from build123d import *

# Parameters (mm, degrees)
SKETCH2_R               = 10.5
BOSS_EXTRUDE1_DEPTH     = 40
SKETCH4_W               = 14
SKETCH4_H               = 22
BOSS_EXTRUDE2_DEPTH     = 38
CUT_EXTRUDE1_DEPTH      = 49.890183064
CUT_EXTRUDE1_DEPTH_BACK = 49.890183064
SKETCH5_W               = 28
SKETCH5_H               = 32.5
SKETCH6_W               = 14
SKETCH6_H               = 38
BOSS_EXTRUDE3_DEPTH     = 40
SKETCH7_W               = 9.5
SKETCH7_H               = 25
BOSS_EXTRUDE4_DEPTH     = 14
BOSS_EXTRUDE5_DEPTH     = 14
SKETCH9_W               = 1
SKETCH9_H               = 30
SKETCH9_H_2             = 31
SKETCH9_H_3             = 20
SKETCH9_H_4             = 15
CUT_EXTRUDE2_DEPTH      = 1
FILLET1_R               = 5
SKETCH10_R              = 12.5
CUT_EXTRUDE3_DEPTH      = 6
SKETCH11_R              = 2.05
CUT_EXTRUDE4_DEPTH      = 116.062756142
SKETCH12_R              = 6
CUT_EXTRUDE5_DEPTH      = 5
CUT_EXTRUDE6_REACH      = 112.061
SKETCH13_R              = 2.05
SKETCH14_R              = 4.5
CUT_EXTRUDE7_DEPTH      = 2
SKETCH15_R              = 1.05
CUT_EXTRUDE8_DEPTH      = 112.975166224
SKETCH17_R              = 2
CUT_EXTRUDE9_DEPTH      = 4


with BuildPart() as part:
    # Sketch2 → Boss-Extrude1 (new body)
    with BuildSketch(Plane.XY):
        Circle(SKETCH2_R)
    extrude(amount=BOSS_EXTRUDE1_DEPTH)

    # Sketch4 → Boss-Extrude2 (add)
    with BuildSketch(Plane.XY.offset(40)):
        with Locations((0, 11)):
            Rectangle(SKETCH4_W, SKETCH4_H)
    extrude(amount=-BOSS_EXTRUDE2_DEPTH)

    # Sketch5 → Cut-Extrude1 (cut, two sides: drawn at the far end of the back side and taken through both)
    with BuildSketch(Plane(origin=(7, 0, 0), x_dir=(0, 0, -1), z_dir=(1, 0, 0)).offset(-CUT_EXTRUDE1_DEPTH_BACK)):
        with Locations((-21, 5.75)):
            Rectangle(SKETCH5_W, SKETCH5_H)
    extrude(amount=CUT_EXTRUDE1_DEPTH + CUT_EXTRUDE1_DEPTH_BACK, mode=Mode.SUBTRACT)


with BuildPart() as cut_extrude1_piece_1:
    # of the separate pieces the step leaves, piece 1, a body of its own (cut_extrude1_pieces)
    add(part.part.solids().sort_by_distance((10.5, 0, 0))[0])



with BuildPart() as cut_extrude1_piece_2:
    # of the separate pieces the step leaves, piece 2, a body of its own (cut_extrude1_pieces)
    add(part.part.solids().sort_by_distance((7, 7.826237921, 40))[0])


with BuildPart() as cut_extrude1_piece_1_1:
    add(cut_extrude1_piece_1.part)

    add(cut_extrude1_piece_2.part)  # Boss-Extrude3 merges Cut-Extrude1 piece 2
    # Sketch6 → Boss-Extrude3 (add)
    with BuildSketch(Plane(origin=(0, 22, 0), x_dir=(1, 0, 0), z_dir=(0, 1, 0))):
        with Locations((0, -21)):
            Rectangle(SKETCH6_W, SKETCH6_H)
    extrude(amount=BOSS_EXTRUDE3_DEPTH)

    # Sketch7 → Boss-Extrude4 (add)
    with BuildSketch(Plane(origin=(7, 0, 0), x_dir=(0, 0, -1), z_dir=(1, 0, 0))):
        Polygon((-52, 42), (-40, 42), (-40, 62), (-40, 67), (-52, 67), align=None)
        Polygon((-40, 67), (-40, 62), (-30.5, 62), (-30.5, 97), (-40, 97), align=None)
        Polygon((-30.5, 97), (-30.5, 62), (-21, 62), (-21, 98), (-21, 102), (-30.5, 102), align=None)
        Polygon((-21, 98), (-21, 62), (-11.5, 62), (-11.5, 87), (-11.5, 98), align=None)
        with Locations((-6.75, 74.5)):
            Rectangle(SKETCH7_W, SKETCH7_H)
    extrude(amount=-BOSS_EXTRUDE4_DEPTH)

    # Sketch8 → Boss-Extrude5 (add)
    with BuildSketch(Plane(origin=(7, 0, 0), x_dir=(0, 0, -1), z_dir=(1, 0, 0))):
        Polygon((-52, 42), (-40, 30), (-40, 42), align=None)
    extrude(amount=-BOSS_EXTRUDE5_DEPTH)

    # Sketch9 → Cut-Extrude2 (cut)
    with BuildSketch(Plane(origin=(7, 0, 0), x_dir=(0, 0, -1), z_dir=(1, 0, 0))):
        with Locations((-30.5, 82)):
            Rectangle(SKETCH9_W, SKETCH9_H)
        with Locations((-21, 82.5)):
            Rectangle(SKETCH9_W, SKETCH9_H_2)
        with Locations((-11.5, 77)):
            Rectangle(SKETCH9_W, SKETCH9_H_3)
        with Locations((-40, 59.5)):
            Rectangle(SKETCH9_W, SKETCH9_H_4)
    extrude(amount=-CUT_EXTRUDE2_DEPTH, mode=Mode.SUBTRACT)

    # Fillet1
    # the kernel refuses this fillet: 5 mm, written as the material it takes off along each edge
    with BuildSketch(Plane(origin=(19.5, 67, 52), x_dir=(0, -1, 0), z_dir=(-1, 0, 0)), Plane(origin=(19.5, 97, 40), x_dir=(0, -1, 0), z_dir=(-1, 0, 0)), Plane(origin=(19.5, 102, 30.5), x_dir=(0, -1, 0), z_dir=(-1, 0, 0)), Plane(origin=(19.5, 98, 11.5), x_dir=(0, 0, 1), z_dir=(-1, 0, 0)), Plane(origin=(19.5, 87, 2), x_dir=(0, 0, 1), z_dir=(-1, 0, 0))) as fillet1_piece_1:
        with BuildLine():
            CenterArc((FILLET1_R, -FILLET1_R), FILLET1_R, 90, 90)
            Line((0, -FILLET1_R), (-FILLET1_R * 0.02, -FILLET1_R))
            Line((-FILLET1_R * 0.02, -FILLET1_R), (-FILLET1_R * 0.02, FILLET1_R * 0.02))
            Line((-FILLET1_R * 0.02, FILLET1_R * 0.02), (FILLET1_R, FILLET1_R * 0.02))
            Line((FILLET1_R, FILLET1_R * 0.02), (FILLET1_R, 0))
        make_face()
    extrude(amount=39, mode=Mode.SUBTRACT)
    with BuildSketch(Plane(origin=(19.247448714, 102, 21), x_dir=(0, 0, 1), z_dir=(-1, 0, 0))) as fillet1_piece_2:
        with BuildLine():
            CenterArc((4.898979486, -5), FILLET1_R, 90, 78.463040967)
            Line((0, -4), (-0.09797959, -3.98))
            ThreePointArc((-0.09797959, -3.98), (-0.1, -2), (-0.1, 0))
            Line((-0.1, 0), (0, 0.1))
            Line((0, 0.1), (4.898979486, 0.1))
            Line((4.898979486, 0.1), (4.898979486, 0))
        make_face()
    extrude(amount=38.494897428, mode=Mode.SUBTRACT)

    # Sketch10 → Cut-Extrude3 (cut)
    with BuildSketch(Plane.ZY.offset(7)):
        with Locations((21, 52)):
            Circle(SKETCH10_R)
    extrude(amount=-CUT_EXTRUDE3_DEPTH, mode=Mode.SUBTRACT)

    # Sketch11 → Cut-Extrude4 (cut, through all)
    with BuildSketch(Plane.ZY.offset(1)):
        with Locations((21, 52)):
            Circle(SKETCH11_R)
    extrude(amount=-CUT_EXTRUDE4_DEPTH, mode=Mode.SUBTRACT)

    # Sketch12 → Cut-Extrude5 (cut)
    with BuildSketch(Plane(origin=(7, 0, 0), x_dir=(0, 0, -1), z_dir=(1, 0, 0))):
        with Locations(Location((-21, 52, 0), (0, 0, 90))):
            Circle(SKETCH12_R)
    extrude(amount=-CUT_EXTRUDE5_DEPTH, mode=Mode.SUBTRACT)

    # Sketch13 → Cut-Extrude6 (cut, up to next)
    with BuildSketch(Plane.XY.offset(40), mode=Mode.PRIVATE) as cut_extrude6_sk1:
        Circle(SKETCH13_R)
    cut_extrude6_tool1 = extrude(cut_extrude6_sk1.sketch, amount=-CUT_EXTRUDE6_REACH, mode=Mode.PRIVATE) & cut_extrude1_piece_1_1.part
    add(cut_extrude6_tool1.solids().sort_by_distance((0, 0, 40))[0], mode=Mode.SUBTRACT)

    # Sketch14 → Cut-Extrude7 (cut)
    with BuildSketch(Plane(origin=(0, 0, 35), x_dir=(-1, 0, 0), z_dir=(0, 0, -1))):
        with Locations(Location((0, 0, 0), (0, 0, 90))):
            Circle(SKETCH14_R)
    extrude(amount=-CUT_EXTRUDE7_DEPTH, mode=Mode.SUBTRACT)

    # Sketch15 → Cut-Extrude8 (cut, through all)
    with BuildSketch(Plane.XY.offset(7)):
        with Locations((-6.062177826, 3.5)):
            Circle(SKETCH15_R)
        with Locations((-6.062177826, -3.5)):
            Circle(SKETCH15_R)
        with Locations((-3.5, -6.062177826)):
            Circle(SKETCH15_R)
        with Locations((0, -7)):
            Circle(SKETCH15_R)
        with Locations((3.5, -6.062177826)):
            Circle(SKETCH15_R)
        with Locations((6.062177826, -3.5)):
            Circle(SKETCH15_R)
        with Locations((7, 0)):
            Circle(SKETCH15_R)
        with Locations((6.062177826, 3.5)):
            Circle(SKETCH15_R)
        with Locations((3.5, 6.062177826)):
            Circle(SKETCH15_R)
        with Locations((0, 7)):
            Circle(SKETCH15_R)
        with Locations((-3.5, 6.062177826)):
            Circle(SKETCH15_R)
        with Locations((-7, 0)):
            Circle(SKETCH15_R)
    extrude(amount=-CUT_EXTRUDE8_DEPTH, mode=Mode.SUBTRACT)

    # Sketch17 → Cut-Extrude9 (cut)
    with BuildSketch(Plane.XY.offset(7)):
        with Locations((0, 7)):
            Circle(SKETCH17_R)
        with Locations((3.5, 6.062177826)):
            Circle(SKETCH17_R)
        with Locations((-3.5, 6.062177826)):
            Circle(SKETCH17_R)
        with Locations((-6.062177826, 3.5)):
            Circle(SKETCH17_R)
        with Locations((-7, 0)):
            Circle(SKETCH17_R)
        with Locations((-6.062177826, -3.5)):
            Circle(SKETCH17_R)
        with Locations((-3.5, -6.062177826)):
            Circle(SKETCH17_R)
        with Locations((0, -7)):
            Circle(SKETCH17_R)
        with Locations((3.5, -6.062177826)):
            Circle(SKETCH17_R)
        with Locations((6.062177826, -3.5)):
            Circle(SKETCH17_R)
        with Locations((7, 0)):
            Circle(SKETCH17_R)
        with Locations((6.062177826, 3.5)):
            Circle(SKETCH17_R)
    extrude(amount=-CUT_EXTRUDE9_DEPTH, mode=Mode.SUBTRACT)


solid = cut_extrude1_piece_1_1.part
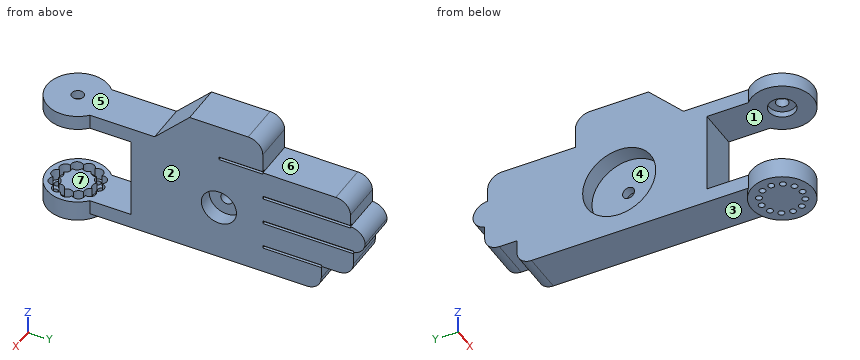
For this review, take the finished solid that the model builds, in its own axes (mm). Face numbers are marked on the shaded views. A direction names the side the tool comes from. Coordinates: 2 decimals unless noted, no trailing zeros. Loops run counter-clockwise (first coordinate to the right, second up) from the corner with the lowest first, then second, coordinate; pieces in that order, holes last. Notation, with made-up numbers: (19.5, -12) -> (65.5, -12) arc R18 ccw to (65.5, 4) -> close; hole circle Ø6 at (22, -21.75). An arc over 180 degrees is marked (long way). Write each question's results on one line, items separated by ' | '.
Q1. Mouldability with a two-part tool opening along Z and no side actions: class the marked faces 1, 2 and 3 as +Z half, -Z half, draft (parallel to the pull), parting line (faces both ways), or undercut.
Taken from the geometry:
face 1: undercut | face 2: draft | face 3: -Z half
Q2. Add section C-C, the plane y = 33. State the section outline as (x, z) points.
Taken from the geometry:
outline: (-7, 2) -> (7, 2) -> (7, 43) -> (-7, 43) -> close
Q3. To check wall thickness, follow line 1 along Z through (x, y) = (4.5, 16); line 2 along Z through (x, y) = (-3, 5); line 3 along Y through (x, z) = (-3.5, 22). State the ranges of each line that lie inside material, in increasing order. Write a range as [from, to].
Taken from the geometry:
line 1: [2, 7], [35, 40] | line 2: [0, 3], [35, 40] | line 3: [22, 39.54], [64.46, 100.13]
Q4. Add section B-B, the plane y = 75.5. State the section outline as (x, z) points, then the cut area to 3 significant figures.
Taken from the geometry:
outline: (-7, 2) -> (7, 2) -> (7, 11) -> (6, 11) -> (6, 12) -> (7, 12) -> (7, 20.5) -> (6, 20.5) -> (6, 21.5) -> (7, 21.5) -> (7, 30) -> (6, 30) -> (6, 31) -> (7, 31) -> (7, 40) -> (-7, 40) -> close | area: 529 mm²
Q5. Add section A-A, the plane z = 5. State the section outline as (x, y) points, then the cut area to 3 significant figures.
Taken from the geometry:
outline: (-7, 7.83) arc R10.5 ccw (long way) to (7, 7.83) -> (7, 86.58) -> (-7, 86.58) -> close; (-5.71, -1.53) arc R2 cw to (-4.18, -4.18) arc R2 cw to (-1.53, -5.71) arc R2 cw to (1.53, -5.71) arc R2 cw to (4.18, -4.18) arc R2 cw to (5.71, -1.53) arc R2 cw to (5.71, 1.53) arc R2 cw to (4.18, 4.18) arc R2 cw to (1.53, 5.71) arc R2 cw to (-1.53, 5.71) arc R2 cw to (-4.18, 4.18) arc R2 cw to (-5.71, 1.53) arc R2 cw to start; hole (-7.35, -1.97) arc R2 ccw to (-5.38, -5.38) arc R2 ccw to (-1.97, -7.35) arc R2 ccw to (1.97, -7.35) arc R2 ccw to (5.38, -5.38) arc R2 ccw to (7.35, -1.97) arc R2 ccw to (7.35, 1.97) arc R2 ccw to (5.38, 5.38) arc R2 ccw to (1.97, 7.35) arc R2 ccw to (-1.97, 7.35) arc R2 ccw to (-5.38, 5.38) arc R2 ccw to (-7.35, 1.97) arc R2 ccw to start | area: 1,280 mm²
Q6. Machinability: for the marked faces 4, 5, 6 and 7, which of the approach directions +Z, -Z, +X, -X, +Y, -Y give a long, thin tool a straight path to every point of the face, cutting with its end or side? Answer none if there is none.
Taken from the geometry:
face 4: -X | face 5: +Z, +X, -X, -Y | face 6: +Z, +X, -X, +Y | face 7: +X, -X, -Y
Q7. For pin 1 Ø1.1 at (x, y) = (6.5, 74.5) entering from +Z; pin 2 Ø2.5 at (x, y) = (-3.5, 6.06) entering from -Z; pin 3 Ø2.5 at (x, y) = (0, 0) entering from +Z; pin 4 Ø1.5 at (y, z) = (41, 39) entering from -X, all flat-tipped, find the tip position at first contact; note any pin that passes through.
Taken from the geometry:
pin 1: z = 40 | pin 2: z = 0 | pin 3: z = 7 | pin 4: x = -7
